For this review, use the dimensioned drawing (mm, ordinates from the lowest corner) and the shaded views. A direction names the side the tool comes from. Round coordinates to 2 decimals unless told otherwise and drop trailing zeros. Loops run counter-clockwise (first coordinate to the right, second up) from the corner with the lowest first, then second, coordinate; pieces in that order, holes last. Notation, with made-up numbers: M 77,78.25 L 127,78.25 A38 ccw 127,117.25 Z; hole C -29.75,56 d9. An arc over 180 degrees is marked long. Answer as a JSON object with one key per item and string values. Group by question number.
Item 1: The part is to be moulded in two halves that separate along Z. For the marked faces 1, 2, 3 and 4, say which applies: +Z half, -Z half, draft (parallel to the pull), parting line (faces both ways), or undercut.
Item 2: Consider section B-B (x = 8). Give the boundary of the cut face in (y, z) (1 decimal).
Item 3: Consider section A-A (y = 6.25). State how many separate pieces and enclosed holes the cut face has, and give its area (3 significant figures).
Item 4: Tool access review of the marked faces 5, 6 and 7: name each direction out of +Z, -Z, +X, -X, +Y, -Y from which nothing blocks a thin tool from reaching the whole face with its end or side.
Item 5: Insertion check: P1, Ø3, axis at x = 20.76, z = 5.12, coming from the -Y side. The pin has a flat end and moves straight along its axis. Give the tip position at first contact, or say it passes through.
Item 6: To check wall thickness, follow line 1 (X direction, y = 2, z = 2.5) (1 decimal); line 2 (X direction, y = 1.25, z = 6) (1 decimal); line 3 (X direction, y = 9, z = 4.75) (1 decimal). State the ranges of each line that lie inside material, in increasing order.
Item 7: Consider section D-D (x = 31). Give the boundary of the cut face in (y, z).
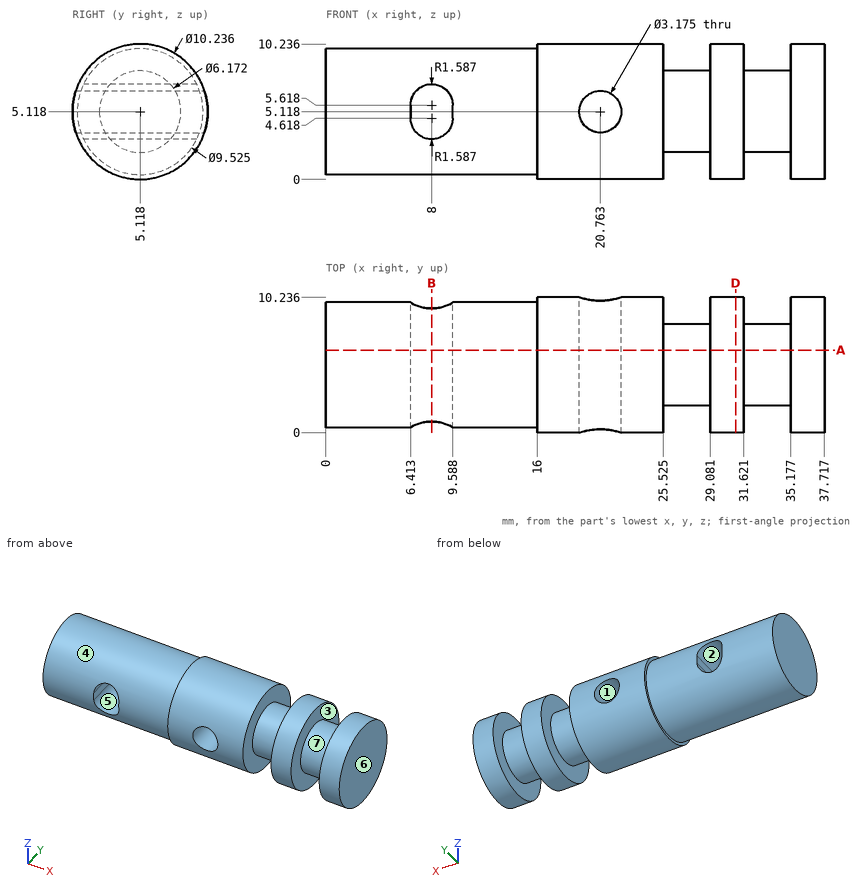
Geometry results:
{
 "1": {"face 1": "undercut", "face 2": "undercut", "face 3": "draft", "face 4": "parting line"},
 "2": {"outline": "M 0.8,3 A4.8 ccw 9.4,3 Z; M 0.8,7.2 L 9.4,7.2 A4.8 ccw Z"},
 "3": {"separate pieces": "1", "enclosed holes": "2", "area": "316 mm^2"},
 "4": {"face 5": "+Y, -Y", "face 6": "+Z, -Z, +X, +Y, -Y", "face 7": "none"},
 "5": {"P1": "passes through"},
 "6": {"line 1": "x = 0 to 25.5, 29.1 to 31.6, 35.2 to 37.7", "line 2": "x = 0 to 6.5, 9.5 to 19.4, 22.1 to 25.5, 29.1 to 31.6, 35.2 to 37.7", "line 3": "x = 0 to 6.4, 9.6 to 19.2, 22.3 to 25.5, 29.1 to 31.6, 35.2 to 37.7"},
 "7": {"outline": "C 5.12,5.12 d10.24"}
}
